from build123d import *

# Parameters (mm, degrees)
PAD_DEPTH    = 3
SKETCH001_R  = 1.5
PAD001_DEPTH = 7.25
SKETCH002_R  = 2.1
POCKET_DEPTH = 2
SKETCH003_R  = 3
PAD002_DEPTH = 3
FILLET_R     = 2.75


with BuildPart() as part:
    # Sketch → Pad (new body)
    with BuildSketch(Plane.XY):
        Polygon((-7.75, 33), (-7.75, -33), (15.75, -33), (15.75, -11.5), (7.75, -11.5), (7.75, 33), (5, 33), (5, 43), (-5, 43), (-5, 33), align=None)
    extrude(amount=PAD_DEPTH)

    # Sketch001 → Pad001 (join, symmetric)
    with BuildSketch(Plane.YZ):
        with Locations((40, 1.5)):
            Circle(SKETCH001_R)
    extrude(amount=PAD001_DEPTH, both=True)

    # Sketch002 (on Face5 of Pad001) → Pocket (cut)
    with BuildSketch(Plane.XY.offset(3)):
        with Locations((4, -23)):
            Circle(SKETCH002_R)
    extrude(amount=-POCKET_DEPTH, mode=Mode.SUBTRACT)

    # Sketch003 (on Face5 of Pocket) → Pad002 (join)
    with BuildSketch(Plane.XY.offset(3)):
        with Locations((0, 23)):
            Circle(SKETCH003_R)
    extrude(amount=PAD002_DEPTH)

    # Fillet
    fillet_edges = [part.edges().sort_by_distance(p)[0] for p in [
        (-3, 23, 6),
    ]]
    fillet(fillet_edges, radius=FILLET_R)


solid = part.part
Verification items for the finished model (mm, model axes). A direction names the side the tool comes from. Give positions to 0.01 mm unless a question says otherwise; leave off trailing zeros. Order: outer loops, then holes, each group sorted by start corner. A loop starts at its lowest first (then second) coordinate and runs counter-clockwise, first axis right, second up. Notation, with made-up numbers: (39, 73.5) -> (69, 73.5) arc R31 cw to (69, 98.5) -> close; hole circle Ø5 at (31.5, -11.75). An arc over 180 degrees is marked (long way). Answer as CSV lines item,"result".
Q1. Sectioned sample at A-A on y = -23. Record the cut outline in (x, z).
Solutions:
outline,"(-7.75, 0) -> (15.75, 0) -> (15.75, 3) -> (6.1, 3) -> (6.1, 1) -> (1.9, 1) -> (1.9, 3) -> (-7.75, 3) -> close"
Q2. Access from +Z, -Z, +X, -X, +Y, -Y to the whole of each face (thin tool, end or side, straight path). Record for faces 4 (the flat face through (6, 33, 1)), 5 (the cylindrical face through (-6.11, 38.5, 1.57)), 6 (the flat face through (7.75, 10, 1)).
Solutions:
face 4,"+Z, -Z, +X"
face 5,"-X"
face 6,"+Z, -Z, +X, +Y"
Q3. Scan lines: probe 1 along Y at (x, z) = (4, 2.2); probe 2 along Z at (x, y) = (-4, 21); probe 3 along Y at (x, z) = (14.25, 1.55). Record each from-to range of solid material in increasing order.
Solutions:
probe 1,"y = -33 to -25.1, -20.9 to 43"
probe 2,"z = 0 to 3"
probe 3,"y = -33 to -11.5"
Q4. Release check for a two-part mould opening along Y. For faces 1 (the flat face through (-5, 42, 1)), 2 (the cylindrical face through (6.14, 38.5, 1.57)), 3 (the flat face through (12, -11.5, 1)) record: +Y half, -Y half, draft (parallel to the pull), parting line (faces both ways), or undercut.
Solutions:
face 1,"draft"
face 2,"undercut"
face 3,"+Y half"
Q5. Sectioned sample at C-C on x = 4. Record the cut outline in (y, z), plus the area to 3 significant figures.
Solutions:
outline,"(-33, 0) -> (43, 0) -> (43, 3) -> (-20.9, 3) -> (-20.9, 1) -> (-25.1, 1) -> (-25.1, 3) -> (-33, 3) -> close"
area,"220 mm²"
Q6. Sectioned sample at B-B on z = 2.2. Record the cut outline in (x, y), plus the area to 3 significant figures.
Solutions:
outline,"(-7.75, -33) -> (15.75, -33) -> (15.75, -11.5) -> (7.75, -11.5) -> (7.75, 33) -> (5, 33) -> (5, 38.67) -> (7.25, 38.67) -> (7.25, 41.33) -> (5, 41.33) -> (5, 43) -> (-5, 43) -> (-5, 41.33) -> (-7.25, 41.33) -> (-7.25, 38.67) -> (-5, 38.67) -> (-5, 33) -> (-7.75, 33) -> close; hole circle Ø4.2 at (4, -23)"
area,"1,290 mm²"
Q7. Sectioned sample at D-D on y = -14.5. Record the cut outline in (x, z).
Solutions:
outline,"(-7.75, 0) -> (15.75, 0) -> (15.75, 3) -> (-7.75, 3) -> close"
Q8. Depth check by flat-ended pin: pin 1 (0.8 mm diameter, centred on x = 7, z = 2, fed in from +Y); pin 2 (4.5 mm diameter, centred on x = 5, y = -23, fed in from +Z); pin 3 (2.5 mm diameter, centred on y = 40.5, z = 1, fed in from +X); pin 4 (2 mm diameter, centred on x = 2, y = 5.5, fed in from -Z). Enter the tip coordinate at first touch or a pass-through.
Solutions:
pin 1,"stops at y = 41.5"
pin 2,"stops at z = 3"
pin 3,"stops at x = 7.25"
pin 4,"stops at z = 0"
